```python
from build123d import *

# Parameters (mm, degrees)
CUT_EXTRUDE2_DEPTH = 15.875


with BuildPart() as part:
    # Sketch3 → Revolve1 (revolve)
    with BuildSketch(Plane.XY):
        with BuildLine():
            Line((0, 15.875), (10.9985175, 9.525002961))
            Line((10.9985175, 9.525002961), (10.9985175, 6.35))
            Line((10.9985175, 6.35), (3.429, 6.35))
            ThreePointArc((3.429, 6.35), (3.159592316, 6.238407684), (3.048, 5.969))
            Line((3.048, 5.969), (3.048, 4.3688))
            Line((3.048, 4.3688), (3.9116, 3.5052))
            Line((3.9116, 3.5052), (3.9116, 0.8636))
            Line((3.9116, 0.8636), (3.048, 0))
            Line((3.048, 0), (0, 0))
            Line((0, 0), (0, 15.875))
        make_face()
    revolve(axis=Axis((0, -1000, 0), (0, 1, 0)))

    # Sketch1 → Cut-Extrude2 (cut)
    with BuildSketch(Plane(origin=(0, 0, 0), x_dir=(1, 0, 0), z_dir=(0, 1, 0))):
        with BuildLine():
            ThreePointArc((-5.499261314, -9.525), (0, -10.998522628), (5.499261314, -9.525))
            Line((5.499261314, -9.525), (-5.499261314, -9.525))
        make_face()
        with BuildLine():
            ThreePointArc((-10.998522628, 0), (-9.525, -5.499261314), (-5.499261314, -9.525))
            Line((-5.499261314, -9.525), (-10.998522628, 0))
        make_face()
        with BuildLine():
            ThreePointArc((5.499261314, -9.525), (9.525, -5.499261314), (10.998522628, 0))
            Line((10.998522628, 0), (5.499261314, -9.525))
        make_face()
        with BuildLine():
            Line((5.499261314, 9.525), (10.998522628, 0))
            ThreePointArc((10.998522628, 0), (9.525, 5.499261314), (5.499261314, 9.525))
        make_face()
        with BuildLine():
            Line((-5.499261314, 9.525), (5.499261314, 9.525))
            ThreePointArc((5.499261314, 9.525), (0, 10.998522628), (-5.499261314, 9.525))
        make_face()
        with BuildLine():
            Line((-10.998522628, 0), (-5.499261314, 9.525))
            ThreePointArc((-5.499261314, 9.525), (-9.525, 5.499261314), (-10.998522628, 0))
        make_face()
    extrude(amount=CUT_EXTRUDE2_DEPTH, mode=Mode.SUBTRACT)


solid = part.part
```
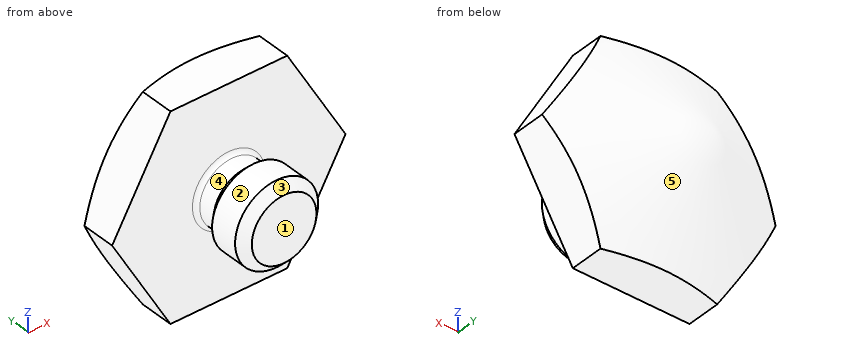
CAD build for the part. Positions are in the model's coordinates, mm. Face numbers are marked on the shaded views. A direction names the side the tool comes from. Coordinates: 2 decimals unless noted, no trailing zeros. Order: outer loops, then holes, each group sorted by start corner. A loop starts at its lowest first (then second) coordinate and runs counter-clockwise, first axis right, second up. Notation, with made-up numbers: (47.5, 25) -> (61.5, 25) arc R14 ccw to (61.5, 52) -> close; hole circle Ø9 at (59.5, -19). An arc over 180 degrees is marked (long way). Use one line per item in the form item = value. Start each with the question number.
1) Drill centre lines: L1, parallel to X at y = 12.75, z = -2.5; L2, parallel to Y at x = -0.75, z = -8.25; L3, parallel to Y at x = 8, z = -0.75. Where is each one in solid material? Low to high. Write a range as [from, to].
2) Band-saw the part on C-C on y = 11.25. Give the cut face in (x, z), then the cut area to 3 significant figures.
3) Pull direction Y, two halves, no side cores. Call the marked faces 3, 4 and 5: +Y half, -Y half, draft (parallel to the pull), parting line (faces both ways), or undercut.
4) Tool access for the marked faces 1 and 2: list every direction of +Z, -Z, +X, -X, +Y, -Y with a clear straight run to the whole face (end or side of a thin tool).
5) Drop flat-ended pins along their axis: pin 1 (6 mm diameter, centred on y = 11, z = 5, fed in from +X); pin 2 (3 mm diameter, centred on x = -7.5, z = 7, fed in from +Y); pin 3 (5 mm diameter, centred on x = 4, y = 2.5, fed in from -Z). Give the stop position or say it passes through.
6) Band-saw the part on B-B on y = 1.25. Give the cut face in (x, z), then the cut area to 3 significant figures.
Entries:
q1.L1 = [-4.8, 4.8]
q1.L2 = [6.35, 11.09]
q1.L3 = [6.35, 11.24]
q2.outline = circle Ø16.02 at (0, 0)
q2.area = 202 mm2
q3.face_3 = -Y half
q3.face_4 = undercut
q3.face_5 = +Y half
q4.face_1 = +Z, -Z, +X, -X, -Y
q4.face_2 = -Y
q5.pin_1 = 9.76
q5.pin_2 = 10.82
q5.pin_3 = -3.61
q6.outline = circle Ø7.82 at (0, 0)
q6.area = 48.1 mm2
